The listing builds one solid part. Answer for the finished solid, in the listing's coordinates (mm). Face numbers are marked on the shaded views. Round coordinates to 2 decimals unless told otherwise and drop trailing zeros. Write each loop counter-clockwise with the first axis right and the second up, starting at its lowest first coordinate (ties: lowest second). Pieces come first, ordered by that corner, then holes.
Item 1: Find section C-C on x = 33. Give the vertices of the cut face in (y, z), then the cut area to 3 significant figures.
Item 2: Each of these flat-tipped pins is pushed along its axis until it touches: pin 1 (1.5 mm diameter, centred on x = 10, z = 1, fed in from -Y); pin 2 (3 mm diameter, centred on x = 28, z = 7.5, fed in from +Y). Where does it stop, or does it pass through?
Item 3: Find section A-A on z = 2.5. Give the vertices of the cut face in (x, y).
Item 4: Find section B-B on y = 30. Give the vertices of the cut face in (x, z), then the cut area to 4 significant figures.
Item 5: For a pull along Y with two mould halves and no side action, classify the marked faces 1, 2 and 3 as +Y half, -Y half, draft (parallel to the pull), parting line (faces both ways), or undercut.
Item 6: Find the intervals of material crossed by probe 1 along X at (y, z) = (39, 1); probe 2 along Y at (x, z) = (50.5, 3.5); probe 3 along X at (y, z) = (68.5, 0.25), in increasing order.
Item 7: Find section D-D on y = 64. Give the vertices of the cut face in (x, z), then the cut area to 3 significant figures.
```python
from build123d import *

# Parameters (mm, degrees)
BOSS_EXTRUDE1_DEPTH     = 10
SKETCH1_3_W             = 25.5
SKETCH1_3_H             = 67
BOSS_EXTRUDE2_DEPTH     = 2.5
CHAMFER1_SIZE           = 10
SKETCH2_W               = 15
SKETCH2_H               = 15
CUT_EXTRUDE1_DEPTH      = 10
CHAMFER2_SIZE           = 5
SKETCH3_W               = 28
SKETCH3_H               = 4
CUT_EXTRUDE2_DEPTH      = 10
FILLET2_R               = 3
FILLET3_R               = 3
CHAMFER3_SIZE           = 10
CUT_EXTRUDE3_DEPTH      = 2.5
CHAMFER4_SIZE           = 13.6
FILLET4_R               = 4
CHAMFER5_SIZE           = 6
CUT_EXTRUDE4_DEPTH      = 135.536240471
CUT_EXTRUDE4_DEPTH_BACK = 2.5
FILLET6_R               = 0.5
SKETCH7_W               = 1.5
SKETCH7_H               = 30
CUT_EXTRUDE5_DEPTH      = 2.5
CHAMFER6_SIZE           = 1.5
FILLET7_R               = 0.5


# Some blends are built 0.0001 mm under size
with BuildPart() as part:
    # Sketch1 → Boss-Extrude1 (new body)
    with BuildSketch(Plane.XY):
        Polygon((56, 67), (56, 69.5), (28, 69.5), (28, 0), (30.5, 0), (30.5, 67), align=None)
        Polygon((56, 120), (56, 69.5), (56, 67), (56, 0), (30.5, 0), (28, 0), (0, 0), (0, 120), (-4, 120), (-4, -4), (60, -4), (60, 120), align=None)
    extrude(amount=BOSS_EXTRUDE1_DEPTH)

    # Sketch1<3> → Boss-Extrude2 (add)
    with BuildSketch(Plane.XY):
        Polygon((28, 69.5), (56, 69.5), (56, 120), (0, 120), (0, 0), (28, 0), align=None)
        with Locations((43.25, 33.5)):
            Rectangle(SKETCH1_3_W, SKETCH1_3_H)
        Polygon((56, 120), (56, 69.5), (56, 67), (56, 0), (30.5, 0), (28, 0), (0, 0), (0, 120), (-4, 120), (-4, -4), (60, -4), (60, 120), align=None)
        Polygon((56, 67), (56, 69.5), (28, 69.5), (28, 0), (30.5, 0), (30.5, 67), align=None)
    extrude(amount=-BOSS_EXTRUDE2_DEPTH)

    # Chamfer1
    chamfer1_edges = [part.edges().sort_by_distance(p)[0] for p in [
        (58, 120, 10),
        (-2, 120, 10),
    ]]
    chamfer(chamfer1_edges, length=CHAMFER1_SIZE)

    # Sketch2 → Cut-Extrude1 (cut)
    with BuildSketch(Plane.XY.offset(10)):
        with Locations((35.5, 62)):
            Rectangle(SKETCH2_W, SKETCH2_H)
    extrude(amount=-CUT_EXTRUDE1_DEPTH, mode=Mode.SUBTRACT)

    # Chamfer2
    chamfer2_edges = [part.edges().sort_by_distance(p)[0] for p in [
        (56, 69.5, 5),
    ]]
    chamfer(chamfer2_edges, length=CHAMFER2_SIZE)

    # Sketch3 → Cut-Extrude2 (cut)
    with BuildSketch(Plane.XY.offset(10)):
        with Locations((14, -2)):
            Rectangle(SKETCH3_W, SKETCH3_H)
    extrude(amount=-CUT_EXTRUDE2_DEPTH, mode=Mode.SUBTRACT)

    # Fillet2
    fillet2_edges = [part.edges().sort_by_distance(p)[0] for p in [
        (28, -4, 5),
    ]]
    fillet(fillet2_edges, radius=FILLET2_R)

    # Fillet3
    fillet3_edges = [part.edges().sort_by_distance(p)[0] for p in [
        (60, -4, 3.75),
    ]]
    fillet(fillet3_edges, radius=FILLET3_R)

    # Chamfer3
    chamfer3_edges = [part.edges().sort_by_distance(p)[0] for p in [
        (-2, -4, 10),
    ]]
    chamfer(chamfer3_edges, length=CHAMFER3_SIZE)

    # Sketch4 → Cut-Extrude3 (cut)
    with BuildSketch(Plane.XY):
        Polygon((36.5, 60.5), (36.5, 61), (37, 61), (50, 61), (50, 6), (36.5, 6), align=None)
        Polygon((10.242640687, 105), (41.25, 105), (50, 96.25), (34.496320344, 80.746320344), align=None)
        Polygon((22, 68.25), (30.253679656, 76.503679656), (6, 100.757359313), (6, 52.25), align=None)
        Polygon((22, 59.764718626), (10.242640687, 48.007359313), (6, 43.764718626), (6, 2), (22, 18), align=None)
    extrude(amount=-CUT_EXTRUDE3_DEPTH, mode=Mode.SUBTRACT)

    # Chamfer4
    # the kernel refuses this chamfer: 13.6 mm, written as the material it adds along each edge
    with BuildSketch(Plane(origin=(50, 6, 0), x_dir=(-0.9996219169112968, -0.0274958766105864, 0), z_dir=(0, 0, -1))) as chamfer4_piece_1:
        Polygon((CHAMFER4_SIZE * 0.999621916911, CHAMFER4_SIZE * 0.0274958766106), (-CHAMFER4_SIZE * 0.0274958766106, CHAMFER4_SIZE * 0.999621916911), (0, 0), align=None)
    extrude(amount=2.5)
    with BuildSketch(Plane(origin=(36.5, 61, 0), x_dir=(-0.027495876610586337, -0.9996219169112968, 0), z_dir=(0, 0, -1))) as chamfer4_piece_2:
        Polygon((CHAMFER4_SIZE * 0.999621916911, -CHAMFER4_SIZE * 0.0274958766106), (-CHAMFER4_SIZE * 0.0274958766106, -CHAMFER4_SIZE * 0.999621916911), (0, 0), align=None)
    extrude(amount=2.5)

    # Fillet4
    fillet4_edges = [part.edges().sort_by_distance(p)[0] for p in [
        (22, 18, -1.25),
        (6, 2, -1.25),
        (6, 43.764718626, -1.25),
        (22, 59.764718626, -1.25),
        (6, 52.25, -1.25),
        (6, 100.757359313, -1.25),
        (30.253679656, 76.503679656, -1.25),
        (41.25, 105, -1.25),
        (50, 96.25, -1.25),
        (34.496320344, 80.746320344, -1.25),
        (10.242640687, 105, -1.25),
        (50, 60.9, -1.25),
        (50, 19.6, -1.25),
        (36.5, 47.4, -1.25),
        (36.5, 6.1, -1.25),
    ]]
    fillet(fillet4_edges, radius=FILLET4_R)

    # Chamfer5
    chamfer5_edges = [part.edges().sort_by_distance(p)[0] for p in [
        (29.25, 54.5, 10),
        (43, 68.25, 10),
    ]]
    chamfer(chamfer5_edges, length=CHAMFER5_SIZE)

    # Sketch6 → Cut-Extrude4 (cut, two sides: drawn at the far end of the back side and taken through both)
    with BuildSketch(Plane.XY.offset(-CUT_EXTRUDE4_DEPTH_BACK)):
        Polygon((34.5, 33.25), (36.5, 33.25), (36.5, 33.75), (36.5, 34.25), (34.5, 34.25), align=None)
        Polygon((36.5, 27.25), (36.5, 27.75), (36.5, 28.25), (34.5, 28.25), (34.5, 27.25), align=None)
        Polygon((50, 33.75), (50, 33.25), (50, 32.75), (52, 32.75), (52, 33.75), align=None)
        Polygon((50, 39.25), (50, 38.75), (52, 38.75), (52, 39.75), (50, 39.75), align=None)
    extrude(amount=CUT_EXTRUDE4_DEPTH + CUT_EXTRUDE4_DEPTH_BACK, mode=Mode.SUBTRACT)

    # Fillet6
    fillet6_edges = [part.edges().sort_by_distance(p)[0] for p in [
        (52, 38.75, -1.25),
        (52, 39.75, -1.25),
        (34.5, 27.25, -1.25),
        (34.5, 28.25, -1.25),
        (34.5, 33.25, -1.25),
        (34.5, 34.25, -1.25),
    ]]
    fillet(fillet6_edges, radius=FILLET6_R - 0.0001)  # a hair under: the kernel refuses the full size

    # Sketch7 → Cut-Extrude5 (cut)
    with BuildSketch(Plane.XY):
        with Locations((27.25, 29.600220455)):
            Rectangle(SKETCH7_W, SKETCH7_H)
    extrude(amount=-CUT_EXTRUDE5_DEPTH, mode=Mode.SUBTRACT)

    # Chamfer6
    chamfer6_edges = [part.edges().sort_by_distance(p)[0] for p in [
        (28, 14.600220455, -1.25),
        (26.5, 44.600220455, -1.25),
    ]]
    chamfer(chamfer6_edges, length=CHAMFER6_SIZE - 0.0001)  # a hair under: the kernel refuses the full size

    # Fillet7
    fillet7_edges = [part.edges().sort_by_distance(p)[0] for p in [
        (52, 32.75, -1.25),
        (52, 33.75, -1.25),
    ]]
    fillet(fillet7_edges, radius=FILLET7_R - 0.0001)  # a hair under: the kernel refuses the full size


solid = part.part
```
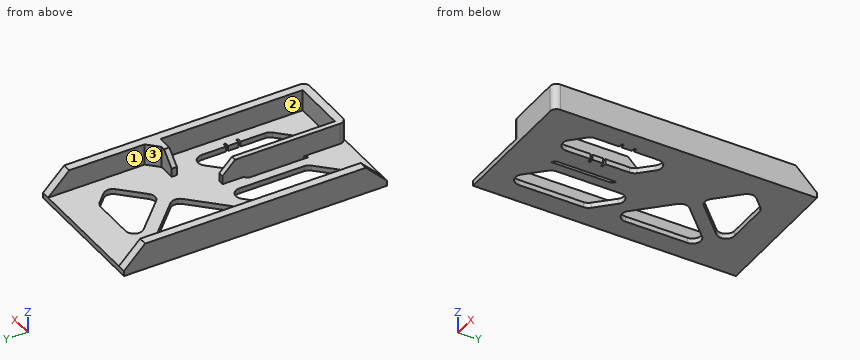
Check values:
1. outline: (-4, -2.5) - (82.69, -2.5) - (82.69, 0) - (0, 0) - (0, 10) - (-4, 10) - close; (105, -2.5) - (120, -2.5) - (120, 0) - (105, 0) - close
1. area: 294 mm2
2. pin 1: passes through
2. pin 2: stops at y = 52.5
3. outline: (-4, -1.5) - (0, -1.5) - (0, 117.5) - (-4, 117.5) - close; (28, -1) arc R3 ccw to (31, -4) - (57, -4) arc R3 ccw to (60, -1) - (60, 117.5) - (56, 117.5) - (56, 74.5) - (51, 69.5) - (43, 69.5) - (43, 67) - (56, 67) - (56, 0) - (30.5, 0) - (30.5, 54.5) - (28, 54.5) - close
4. outline: (-4, -2.5) - (6, -2.5) - (6, 0) - (0, 0) - (0, 10) - (-4, 10) - close; (22, -2.5) - (26.5, -2.5) - (26.5, 0) - (22, 0) - close; (28, -2.5) - (36.5, -2.5) - (36.5, 0) - (30.5, 0) - (30.5, 10) - (28, 10) - close; (50, -2.5) - (60, -2.5) - (60, 10) - (56, 10) - (56, 0) - (50, 0) - close
4. area: 187.5 mm2
5. face 1: draft
5. face 2: undercut
5. face 3: +Y half
6. probe 1: x = -4 to 0, 28 to 30.5, 56 to 60
6. probe 2: y = -4 to 0, 67 to 69.5
6. probe 3: x = -4 to 0, 43 to 60
7. outline: (-4, -2.5) - (6, -2.5) - (6, 0) - (0, 0) - (0, 10) - (-4, 10) - close; (17.75, -2.5) - (60, -2.5) - (60, 10) - (56, 10) - (56, 0) - (17.75, 0) - close
7. area: 211 mm2
